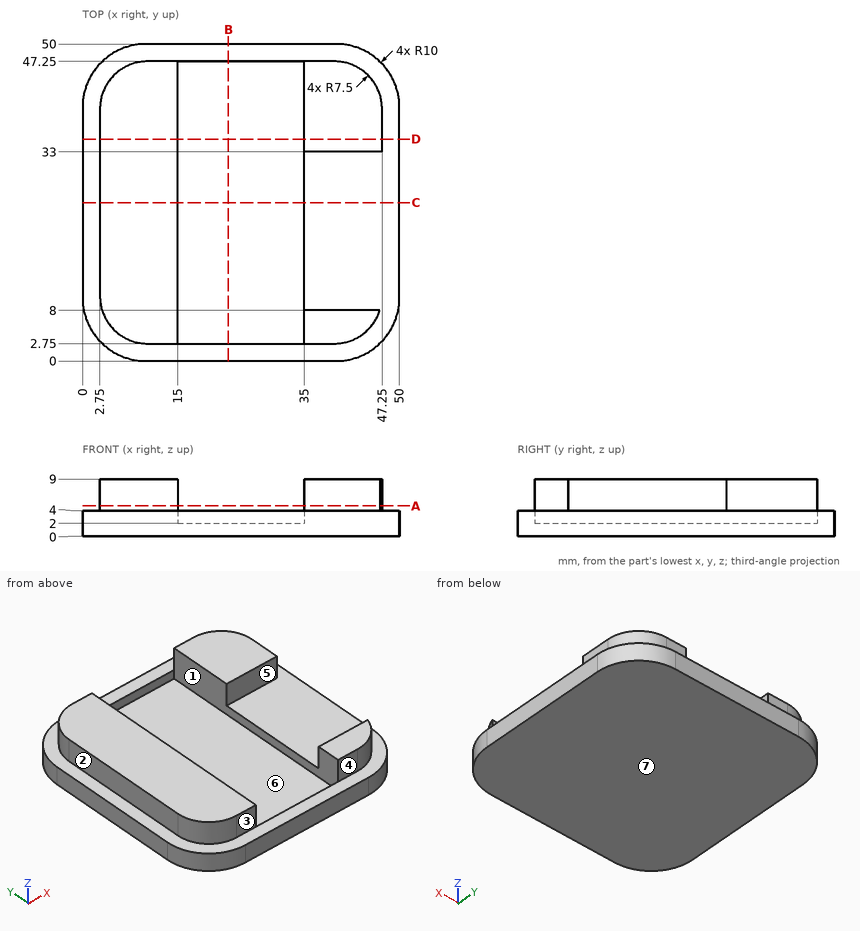
Study the drawing (mm; zero at the part's minimum x, y, z) and answer. A direction names the side the tool comes from. Coordinates: 2 decimals unless noted, no trailing zeros. Loops run counter-clockwise (first coordinate to the right, second up) from the corner with the lowest first, then second, coordinate; pieces in that order, holes last. Notation, with made-up numbers: (-28, -15) -> (0, -15) arc R31 cw to (0, 23) -> close; hole circle Ø2 at (74, -37). An arc over 180 degrees is marked (long way). Answer as CSV lines item,"result".
1) For the marked faces 1, 2 and 3, determine the directions among +Z, -Z, +X, -X, +Y, -Y from which every point of the face is accessible in a straight line to the end or side of a thin tool.
A:
face 1,"+Z"
face 2,"+Z, -X, +Y, -Y"
face 3,"+Z, +X, -X, -Y"
2) The part is cut by section A-A (z = 4.75). Give the vertices of the cut face in (x, y).
A:
outline,"(2.75, 10.25) arc R7.5 ccw to (10.25, 2.75) -> (15, 2.75) -> (15, 47.25) -> (10.25, 47.25) arc R7.5 ccw to (2.75, 39.75) -> close; (35, 2.75) -> (39.75, 2.75) arc R7.5 ccw to (46.9, 8) -> (35, 8) -> close; (35, 33) -> (47.25, 33) -> (47.25, 39.75) arc R7.5 ccw to (39.75, 47.25) -> (35, 47.25) -> close"
3) For a pull along Y with two mould halves and no side action, classify the marked faces 4, 5, 6 and 7 as released by +Y, released by -Y, zero draft, split by the parting line, or undercut.
A:
face 4,"released by -Y"
face 5,"undercut"
face 6,"undercut"
face 7,"zero draft"
4) Straight lines are drawn through the part: probe 1 along X at (y, z) = (38, 7.5); probe 2 along X at (y, z) = (13.5, 3.25); probe 3 along Y at (x, z) = (16.5, 2.5). For each, find the intervals that lie inside material, in ascending order.
A:
probe 1,"x = 2.75 to 15, 35 to 47.25"
probe 2,"x = 0 to 15, 35 to 50"
probe 3,"y = 0 to 2.75, 47.25 to 50"
5) Flat-ended cylindrical pins translate along their axes: pin 1 (1 mm diameter, centred on y = 9, z = 4, fed in from +X); pin 2 (4 mm diameter, centred on x = 40, z = 7, fed in from +Y); pin 3 (22 mm diameter, centred on x = 29, y = 25.5, fed in from +Z); pin 4 (15 mm diameter, centred on x = 34, y = 21.5, fed in from +Z). Find the tip coordinate at first contact, or state that the pin passes through.
A:
pin 1,"stops at x = 49.99"
pin 2,"stops at y = 47.25"
pin 3,"stops at z = 9"
pin 4,"stops at z = 4"
6) The part is cut by section B-B (x = 23). Give the vertices of the cut face in (y, z), and give its area (3 significant figures).
A:
outline,"(0, 0) -> (50, 0) -> (50, 4) -> (47.25, 4) -> (47.25, 2) -> (2.75, 2) -> (2.75, 4) -> (0, 4) -> close"
area,"111 mm²"
7) The part is cut by section C-C (y = 25). Give the vertices of the cut face in (x, z), and give its area (3 significant figures).
A:
outline,"(0, 0) -> (50, 0) -> (50, 4) -> (35, 4) -> (35, 2) -> (15, 2) -> (15, 9) -> (2.75, 9) -> (2.75, 4) -> (0, 4) -> close"
area,"221 mm²"
8) The part is cut by section D-D (y = 35). Give the vertices of the cut face in (x, z).
A:
outline,"(0, 0) -> (50, 0) -> (50, 4) -> (47.25, 4) -> (47.25, 9) -> (35, 9) -> (35, 2) -> (15, 2) -> (15, 9) -> (2.75, 9) -> (2.75, 4) -> (0, 4) -> close"
